Verification items for this drawing (mm, ordinates from the low corner). Coordinates: 2 decimals unless noted, no trailing zeros. Write each loop counter-clockwise with the first axis right and the second up, starting at its lowest first coordinate (ties: lowest second). Pieces come first, ordered by that corner, then holes. Notation, with made-up numbers: M 84,24 L 112,24 A22 cw 112,48 Z; hole C 84,-2.75 d11. An arc over 180 degrees is marked long. Put each result on its own line as item: value. Start each with the question number.
1) Gauge pin test, flat end, axial feed: pin 1 (1 mm diameter, centred on y = 1.5, z = 20, fed in from -X). Record the tip position at first contact, or that the pin passes through.
2) Cross-section at A-A on z = 46. Count the separate pieces of the cut face and the enclosed holes in it.
3) Cross-section at C-C on z = 12. Record the cut outline in (x, y) (1 decimal).
4) Scan lines: line 1 along X through (y, z) = (2.1, 15); line 2 along Z through (x, y) = (23, 1); line 3 along X through (y, z) = (2.5, 35.5). Record each from-to range of solid material in increasing order.
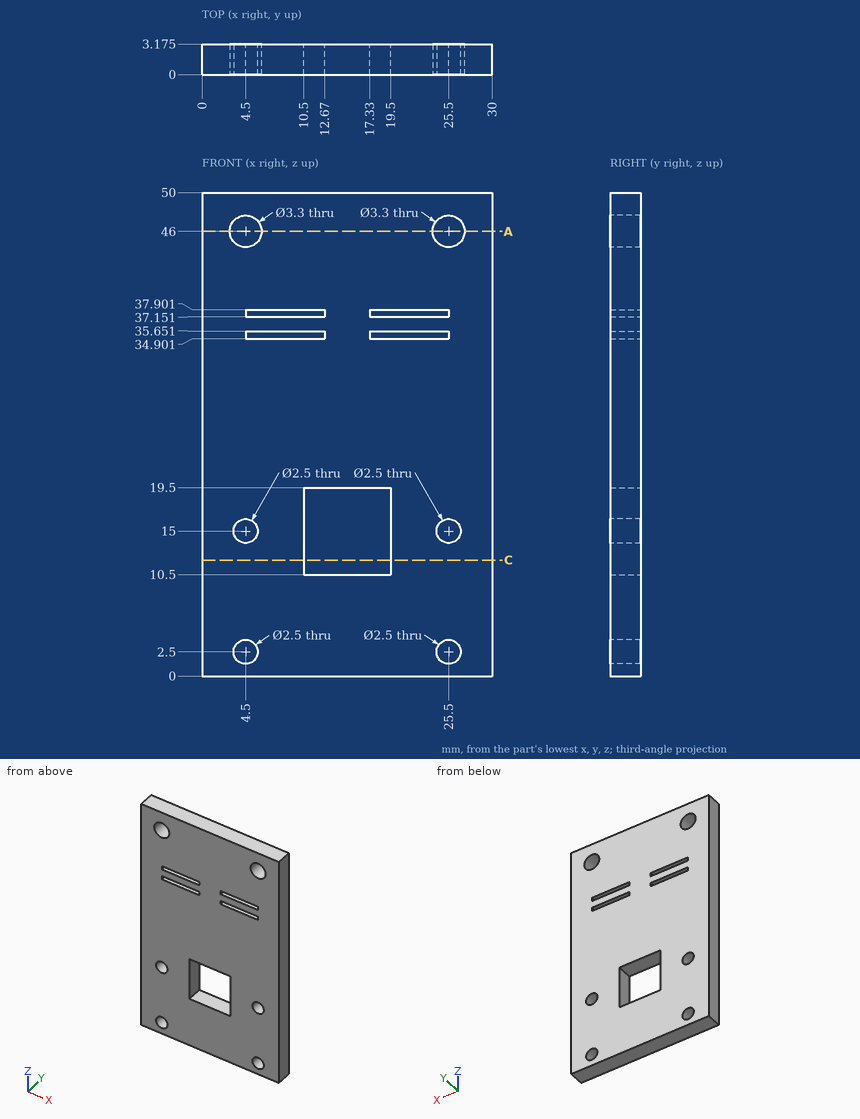
Answer key:
1. pin 1: stops at x = 0
2. separate pieces: 3
2. enclosed holes: 0
3. outline: M 0,0 L 10.5,0 L 10.5,3.2 L 0,3.2 Z; M 19.5,0 L 30,0 L 30,3.2 L 19.5,3.2 Z
4. line 1: x = 0 to 3.25, 5.75 to 10.5, 19.5 to 24.25, 26.75 to 30
4. line 2: z = 0 to 34.9, 35.65 to 37.15, 37.9 to 50
4. line 3: x = 0 to 4.5, 12.67 to 17.33, 25.5 to 30
